```python
from build123d import *

# Parameters (mm, degrees)
SKETCH1_R           = 2.75
SKETCH1_R_2         = 1.5
BOSS_EXTRUDE1_DEPTH = 4


with BuildPart() as part:
    # Sketch1 → Boss-Extrude1 (new body)
    with BuildSketch(Plane(origin=(0, 0, 0), x_dir=(1, 0, 0), z_dir=(0, 1, 0))):
        with BuildLine():
            Line((-5.42452127, 18.55232243), (-6.592163913, 0.424614729))
            ThreePointArc((-6.592163913, 0.424614729), (0.204408635, -6.602661572), (6.553274043, 0.831578043))
            Line((6.553274043, 0.831578043), (5.554165127, 8.705083814))
            ThreePointArc((5.554165127, 8.705083814), (6.283820074, 11.556382789), (8.766792184, 13.136620645))
            Line((8.766792184, 13.136620645), (26.80965439, 16.607175604))
            Line((26.80965439, 16.607175604), (46.521475319, 15.034505243))
            ThreePointArc((46.521475319, 15.034505243), (49.9462455, 17.999804862), (46.927651625, 21.377695275))
            Line((46.927651625, 21.377695275), (0.262324785, 23.632347033))
            ThreePointArc((0.262324785, 23.632347033), (-3.621288531, 22.256778313), (-5.42452127, 18.55232243))
        make_face()
        with Locations(Location((0, 0, 0), (0, 0, 270))):
            Circle(SKETCH1_R, mode=Mode.SUBTRACT)
        with Locations(Location((46.774261136, 18.202917946, 0), (0, 0, 270))):
            Circle(SKETCH1_R_2, mode=Mode.SUBTRACT)
    extrude(amount=BOSS_EXTRUDE1_DEPTH)


solid = part.part
```
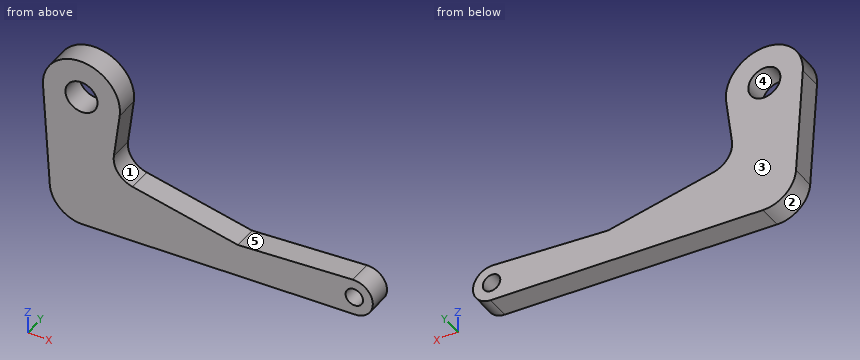
Could you check a few things on this model? Use its own coordinates, in mm. Face numbers are marked on the shaded views. A direction names the side the tool comes from. Coordinates: 2 decimals unless noted, no trailing zeros. Loops run counter-clockwise (first coordinate to the right, second up) from the corner with the lowest first, then second, coordinate; pieces in that order, holes last.
1) Imagine slicing it at C-C (x = -2). List the corners of the cut face in (y, z) for me.
Reported:
outline: (0, -23.26) - (4, -23.26) - (4, -1.89) - (0, -1.89) - close; (0, 1.89) - (4, 1.89) - (4, 6.3) - (0, 6.3) - close
2) Imagine slicing it at A-A (z = 1). List the corners of the cut face in (x, y) for me, and give its area (3 significant figures).
Reported:
outline: (-6.53, 0) - (-2.56, 0) - (-2.56, 4) - (-6.53, 4) - close; (2.56, 0) - (6.53, 0) - (6.53, 4) - (2.56, 4) - close
area: 31.7 mm2
3) Imagine slicing it at B-B (y = 3.2). List the corners of the cut face in (x, z) for me.
Reported:
outline: (-6.59, -0.42) - (-5.42, -18.55) arc R5.44 ccw to (0.26, -23.63) - (46.93, -21.38) arc R3.18 ccw (long way) to (46.52, -15.03) - (26.81, -16.61) - (8.77, -13.14) arc R4 cw to (5.55, -8.71) - (6.55, -0.83) arc R6.61 ccw (long way) to start; hole circle Ø5.5 at (0, 0); hole circle Ø3 at (46.77, -18.2)
4) Thinking about a two-plate mould opening in Z: for the marked faces 1, 2 and 3, which applies, released by +Z, released by -Z, zero draft, split by the parting line, or undercut?
Reported:
face 1: undercut
face 2: released by -Z
face 3: zero draft
5) Will these pins go through, and if not, where does the flat tip stop? pin 1 Ø2 at (y, z) = (2, -8) entering from -X; pin 2 Ø1 at (x, y) = (33, 3) entering from +Z; pin 3 Ø1.5 at (x, y) = (36.5, 3) entering from +Z.
Reported:
pin 1: stops at x = -6.17
pin 2: stops at z = -16.07
pin 3: stops at z = -15.77
6) Please list where these lines run through material, in increasing order: line 1 along X through (y, z) = (0.4, 0); line 2 along X through (y, z) = (1.4, 3); line 3 along Z through (x, y) = (4.5, 2.25).
Reported:
line 1: x = -6.61 to -2.75, 2.75 to 6.61
line 2: x = -5.89 to 5.89
line 3: z = -23.43 to 4.84
7) Which directions (+Z, -Z, +X, -X, +Y, -Y) give clear straight access to the entire face, cutting with the end or side of a thin tool? Please do the marked faces 4 and 5.
Reported:
face 4: +Y, -Y
face 5: +Z, +Y, -Y
8) Imagine slicing it at D-D (x = 19). List the corners of the cut face in (y, z) for me, and give its area (3 significant figures).
Reported:
outline: (0, -22.73) - (4, -22.73) - (4, -15.1) - (0, -15.1) - close
area: 30.5 mm2
